Build history of the part. All positions in model axes, mm. Face numbers are marked on the shaded views. A direction names the side the tool comes from. Round coordinates to 2 decimals unless told otherwise and drop trailing zeros. Order: outer loops, then holes, each group sorted by start corner. A loop starts at its lowest first (then second) coordinate and runs counter-clockwise, first axis right, second up. Notation, with made-up numbers: (58.5, 36) -> (111.5, 36) arc R20 cw to (111.5, 71) -> close; hole circle Ø7 at (74.5, 20). An arc over 180 degrees is marked (long way). Answer as a JSON object with one key per item and string values.
Autodesk Inventor part; units mm, degrees
ref_plane "Work Plane1" through (0, 10, 0) normal (0, 1, 0) x (1, 0, 0)
ref_plane "YZ Plane" through (0, 0, 0) normal (1, 0, 0) x (0, 1, 0)
ref_plane "XZ Plane" through (0, 0, 0) normal (0, 1, 0) x (-1, 0, 0)
sketch "Sketch1" plane through (0, 0, 0) normal (0, 0, 1) x (1, 0, 0)
  line L0 (-32.5, 15) -> (32.5, 15)
  line L1 (32.5, 15) -> (32.5, -15)
  line L2 (-32.5, -15) -> (-32.5, 15)
  line L3 (-32.5, 15) -> (32.5, -15) construction
  line L4 (32.5, 15) -> (-32.5, -15) construction
  line L5 (-22.5, 15) -> (11.5921, 15) construction
  line L6 (-22.5, -15) -> (-49.5, -15)
  line L7 (-52.5, -18) -> (-52.5, -65)
  line L8 (-52.5, -65) -> (-65.5, -65)
  line L9 (-65.5, -65) -> (-65.5, -6.6898)
  line L10 (-64.0549, -4.1242) -> (-32.5, 15)
  arc A0 (-64.0549, -4.1242) -> (-65.5, -6.6898) centre (-62.5, -6.6898) ccw
  arc A1 (-49.5, -15) -> (-52.5, -18) centre (-49.5, -18) ccw
  line L11 (32.5, -15) -> (22.5, -15)
  line L12 (32.5, -15) -> (49.5, -15)
  line L13 (52.5, -18) -> (52.5, -45)
  line L14 (52.5, -45) -> (65.5, -45)
  line L15 (65.5, -45) -> (65.5, -6.6898)
  line L16 (64.0549, -4.1242) -> (32.5, 15)
  arc A2 (65.5, -6.6898) -> (64.0549, -4.1242) centre (62.5, -6.6898) ccw
  arc A3 (52.5, -18) -> (49.5, -15) centre (49.5, -18) ccw
  line L17 (-22.5, -15) -> (22.5, -15)
  point P0 (0, 0)
  point P1 (-22.5, -2.0461)
  point P2 (-52.5, -15)
  point P3 (-65.5, -5)
  point P4 (52.5, -15)
  point P5 (65.5, -5)
  dimension "d0" = 65
  dimension "d1" = 30
  dimension "d3" = 10
  dimension "d4" = 30
  dimension "d5" = 50
  dimension "d6" = 13
  dimension "d7" = 60
  dimension "d8" = 3
  dimension "d10" = 20
  dimension "d11" = 30
  dimension "d12" = 13
  dimension "d13" = 40
  dimension "d14" = 3
extrude "Extrusion1" add sketch "Sketch1" along normal mid plane 50
sketch "Sketch2" plane through (-32.5, 15, 25) normal (0, 1, 0) x (1, 0, 0)
  circle A0 centre (32.5, 25) radius 32.5
  dimension "d17" = 65
extrude "Extrusion2" add sketch "Sketch2" along normal blind 5 and the other way blind 40
sketch "Sketch3" plane through (0, 20, 0) normal (0, 1, 0) x (1, 0, 0)
  circle A0 centre (0, 0) radius 27.5
  dimension "d22" = 55
sketch "Sketch4" plane through (0, 20, 0) normal (0, 1, 0) x (1, 0, 0)
  point P0 (0, 0)
extrude "Extrusion3" cut sketch "Sketch3" against normal through all
ref_plane "Work Plane1" through (0, 10, 0) normal (0, 1, 0) x (1, 0, 0)
sketch "Sketch5" plane through (0, 10, 0) normal (0, 1, 0) x (1, 0, 0)
  circle A0 centre (0, 0) radius 27.5
  circle A1 centre (0, 0) radius 22.5
  dimension "d26" = 55
  dimension "d27" = 45
extrude "Extrusion4" add sketch "Sketch5" against normal blind 25
sketch "Sketch6" plane through (-65.5, -65, 25) normal (-1, 0, 0) x (0, 0, 1)
  circle A0 centre (-24.7708, 20) radius 5
  line L0 (-50, 0) -> (-50, 58.3102)
  line L1 (2.5, 40) -> (-52.5, 40)
  line L2 (-50, 0) -> (0.2292, 0)
  line L3 (0.2292, 0) -> (0.2292, 40)
  line L4 (0.2292, 40) -> (-50, 40)
  line L5 (-50, 40) -> (-50, 0)
  point P0 (-25, 65)
  dimension "d30" = 10
  dimension "d31" = 20
  dimension "d33" = 25
extrude "Extrusion5" cut sketch "Sketch6" against normal blind 25 contours A0
sketch "Sketch7" plane through (65.5, -45, 25) normal (1, 0, 0) x (0, 0, -1)
  circle A0 centre (25, 20) radius 5
  line L0 (50, 0) -> (0, 0)
  line L1 (50, 38.3102) -> (50, 0)
  point P0 (25, 45)
  dimension "d36" = 10
  dimension "d37" = 20
  dimension "d38" = 25
extrude "Extrusion6" cut sketch "Sketch7" against normal blind 20
sketch "Sketch8" plane through (0, 0, -25) normal (0, 0, -1) x (-1, 0, 0)
  line L0 (32.5, 15) -> (64.0549, -4.1242)
  line L1 (32.5, 15) -> (32.5, 3)
  line L2 (32.5, 3) -> (52.4996, 2.879)
  point P0 (0, 0)
  dimension "d41" = 12
  dimension "d42" = 20
extrude "Extrusion7" cut sketch "Sketch8" against normal blind 15
sketch "Sketch9" plane through (-52.4996, 2.879, -10) normal (-0.006, 1, 0) x (1, 0.006, 0)
  circle A0 centre (5, 7.5) radius 2.5
  circle A1 centre (15, 7.5) radius 2.5
  line L0 (0, 0) -> (0, 15)
  line L1 (20.0726, 15) -> (20.0726, 0)
  line L2 (0, 15) -> (20, 15)
  point P0 (52.4813, -10)
  dimension "d45" = 5
  dimension "d46" = 5
  dimension "d48" = 10
  dimension "d49" = 5
  dimension "d51" = 7.5
  dimension "d52" = 7.5
extrude "Extrusion8" cut sketch "Sketch9" against normal blind 25
sketch "Sketch10" plane through (-49.5, -15, -25) normal (0, -1, 0) x (1, 0, 0)
  line L0 (17, 0) -> (17, 15)
  line L1 (-2.9996, 15) -> (17, 15)
  line L2 (17, 0) -> (-1, 0)
  line L3 (-1, 0) -> (-1, 15)
  line L4 (-1, 15) -> (17, 15)
  line L5 (17, 15) -> (17, 0)
  point P0 (49.5, 25)
  dimension "d55" = 18
extrude "Extrusion9" cut sketch "Sketch10" against normal blind 5
equation "\"d52\" = d51"
properties part number "upright2025"
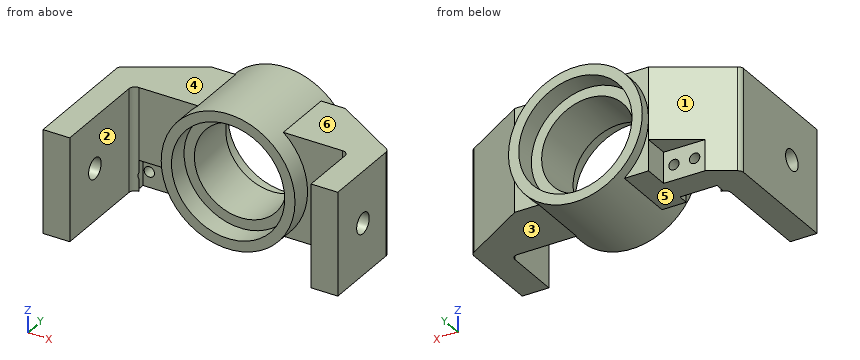
1) Pull direction X, two halves, no side cores. Call the marked faces 1, 2 and 3: pulls with the +X half, pulls with the -X half, needs draft (parallel to the pull), parting line crosses it, or undercut.
Checked values:
{"face 1": "pulls with the -X half", "face 2": "undercut", "face 3": "needs draft"}
2) Which spindle directions (+Z, -Z, +X, -X, +Y, -Y) get a long thin tool onto all of the face, cutting with end or side? Do the marked faces 4, 5 and 6. Say none if no direction does.
Checked values:
{"face 4": "+Z, -X, +Y, -Y", "face 5": "-Z, -X, +Y, -Y", "face 6": "+Z, +X, +Y, -Y"}
3) Flat gauge pins, fed straight in: pin 1 Ø8 at (y, z) = (-45, 0.23) entering from -X; pin 2 Ø12 at (x, y) = (-51.5, -16) entering from +Z; pin 3 Ø1.5 at (x, z) = (26, 5.5) entering from +Y. Where does each tip first touch, or does it go through?
Checked values:
{"pin 1": "stops at x = 52.5", "pin 2": "stops at z = 25", "pin 3": "stops at y = 10"}
4) Probe L1, parallel to Z at x = 0, y = -20; L2, parallel to X at y = -27.5, z = -5; L3, parallel to Z at x = -28.5, y = 1.5. List the from-to ranges inside material, lowest first. Write a range as from..to.
Checked values:
{"L1": "z = -32.5..-27.5, 27.5..32.5", "L2": "x = -65.5..-52.5, 52.5..65.5", "L3": "z = -25..25"}
5) Cut at D-D, the plane x = 17.5. Give the cut face in (y, z).
Checked values:
{"outline": "(-25, -27.39) -> (20, -27.39) -> (20, -21.21) -> (10, -21.21) -> (10, -14.14) -> (-15, -14.14) -> (-15, -21.21) -> (-25, -21.21) -> close; (-25, 21.21) -> (-15, 21.21) -> (-15, 14.14) -> (10, 14.14) -> (10, 21.21) -> (20, 21.21) -> (20, 27.39) -> (-25, 27.39) -> close"}
6) Cut at A-A, the plane x = 0. Give the cut face in (y, z), plus the area to 3 significant figures.
Checked values:
{"outline": "(-25, -32.5) -> (20, -32.5) -> (20, -27.5) -> (10, -27.5) -> (10, -22.5) -> (-15, -22.5) -> (-15, -27.5) -> (-25, -27.5) -> close; (-25, 27.5) -> (-15, 27.5) -> (-15, 22.5) -> (10, 22.5) -> (10, 27.5) -> (20, 27.5) -> (20, 32.5) -> (-25, 32.5) -> close", "area": "700 mm²"}
